Read the model definition and answer for the solid it produces. Units are mm, in the model's axes. Face numbers are marked on the shaded views. A direction names the side the tool comes from. Give positions to 0.01 mm unless a question says otherwise; leave off trailing zeros. Order: outer loops, then holes, each group sorted by start corner. A loop starts at its lowest first (then second) coordinate and runs counter-clockwise, first axis right, second up.
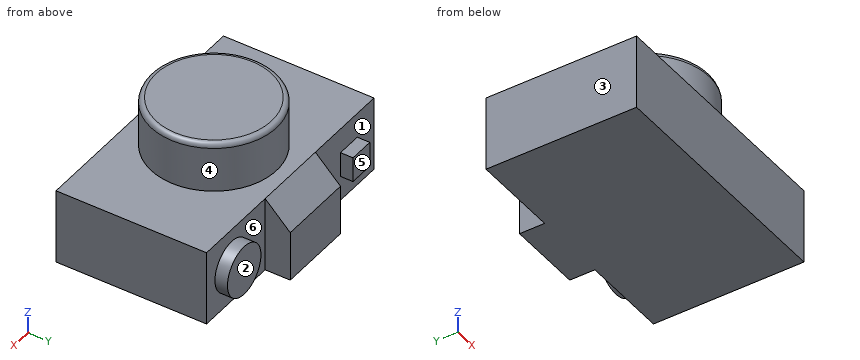
```python
from build123d import *

# Parameters (mm, degrees)
SKETCH2_W           = 100
SKETCH2_H           = 60
BOSS_EXTRUDE1_DEPTH = 30
SKETCH4_R           = 25
BOSS_EXTRUDE2_DEPTH = 20
SKETCH6_R           = 10
SKETCH6_W           = 10
SKETCH6_H           = 10
BOSS_EXTRUDE3_DEPTH = 5
SKETCH8_W           = 30
SKETCH8_H           = 30
BOSS_EXTRUDE4_DEPTH = 10
CHAMFER2_SIZE       = 10
FILLET1_R           = 2


with BuildPart() as part:
    # Sketch2 → Boss-Extrude1 (new body)
    with BuildSketch(Plane.XY):
        with Locations((2.802056555, -2.390745501)):
            Rectangle(SKETCH2_W, SKETCH2_H)
    extrude(amount=BOSS_EXTRUDE1_DEPTH)

    # Sketch4 → Boss-Extrude2 (add)
    with BuildSketch(Plane.XY.offset(30)):
        with Locations((3.165713288, -2.608939541)):
            Circle(SKETCH4_R)
    extrude(amount=BOSS_EXTRUDE2_DEPTH)

    # Sketch6 → Boss-Extrude3 (add)
    with BuildSketch(Plane(origin=(0, 27.609254499, 0), x_dir=(1, 0, 0), z_dir=(0, 1, 0))):
        with Locations((37.802056555, -15)):
            Circle(SKETCH6_R)
        with Locations((-32.197943445, -15)):
            Rectangle(SKETCH6_W, SKETCH6_H)
    extrude(amount=BOSS_EXTRUDE3_DEPTH)

    # Sketch8 → Boss-Extrude4 (add)
    with BuildSketch(Plane(origin=(0, 27.609254499, 0), x_dir=(1, 0, 0), z_dir=(0, 1, 0))):
        with Locations((2.802056555, -15)):
            Rectangle(SKETCH8_W, SKETCH8_H)
    extrude(amount=BOSS_EXTRUDE4_DEPTH)

    # Chamfer2
    chamfer2_edges = [part.edges().sort_by_distance(p)[0] for p in [
        (2.802056555, 37.609254499, 30),
    ]]
    chamfer(chamfer2_edges, length=CHAMFER2_SIZE)

    # Fillet1
    fillet1_edges = [part.edges().sort_by_distance(p)[0] for p in [
        (-21.834286712, -2.608939541, 50),
    ]]
    fillet(fillet1_edges, radius=FILLET1_R)


solid = part.part
```
1) For a pull along X with two mould halves and no side action, classify the marked faces 1, 2 and 3 as released by +X, released by -X, zero draft, split by the parting line, or undercut.
Final values:
face 1: undercut
face 2: zero draft
face 3: released by -X
2) The part is cut by section A-A on x = -34. Determine the outline of the cut face in (y, z), and give its area (3 significant figures).
Final values:
outline: (-32.39, 0) - (27.61, 0) - (27.61, 10) - (32.61, 10) - (32.61, 20) - (27.61, 20) - (27.61, 30) - (-32.39, 30) - close
area: 1,850 mm2
3) Given pin 1 (2.5 mm diameter, centred on x = -34.5, y = 29, fed in from -Z); pin 2 (5.5 mm diameter, centred on x = -34, y = 30.5, fed in from +Z); pin 3 (11 mm diameter, centred on x = -31.5, z = 14.5, fed in from +Y), each flat-ended and moving along its own axis, determine where each tip first touches the part or whether it passes through.
Final values:
pin 1: stops at z = 10
pin 2: stops at z = 20
pin 3: stops at y = 32.61
4) The part is cut by section C-C on z = 6.5. Determine the outline of the cut face in (x, y), and give its area (3 significant figures).
Final values:
outline: (-47.2, -32.39) - (52.8, -32.39) - (52.8, 27.61) - (43.07, 27.61) - (43.07, 32.61) - (32.53, 32.61) - (32.53, 27.61) - (17.8, 27.61) - (17.8, 37.61) - (-12.2, 37.61) - (-12.2, 27.61) - (-47.2, 27.61) - close
area: 6,350 mm2
5) Consider L1, parallel to X at y = 28.5, z = 18; L2, parallel to Y at x = 20, z = 7; L3, parallel to Z at x = 24, y = 19. Determine where each line is inside the solid, lowest interval first.
Final values:
L1: x = -37.2 to -27.2, -12.2 to 17.8, 28.26 to 47.34
L2: y = -32.39 to 27.61
L3: z = 0 to 30
6) A tool of negligible diameter and unlimited length cuts with its end or side. For the marked faces 4, 5 and 6, from which of +Z, -Z, +X, -X, +Y, -Y can it reach the whole face along a straight path? Write none if from no direction.
Final values:
face 4: +Z
face 5: +Z, -Z, -X, +Y
face 6: +Y
7) The part is cut by section D-D on x = 40. Determine the outline of the cut face in (y, z).
Final values:
outline: (-32.39, 0) - (27.61, 0) - (27.61, 5.24) - (32.61, 5.24) - (32.61, 24.76) - (27.61, 24.76) - (27.61, 30) - (-32.39, 30) - close
8) The part is cut by section B-B on y = 31. Determine the outline of the cut face in (x, z), and give its area (3 significant figures).
Final values:
outline: (-37.2, 10) - (-27.2, 10) - (-27.2, 20) - (-37.2, 20) - close; (-12.2, 0) - (17.8, 0) - (17.8, 26.61) - (-12.2, 26.61) - close; circle Ø20 at (37.8, 15)
area: 1,210 mm2
